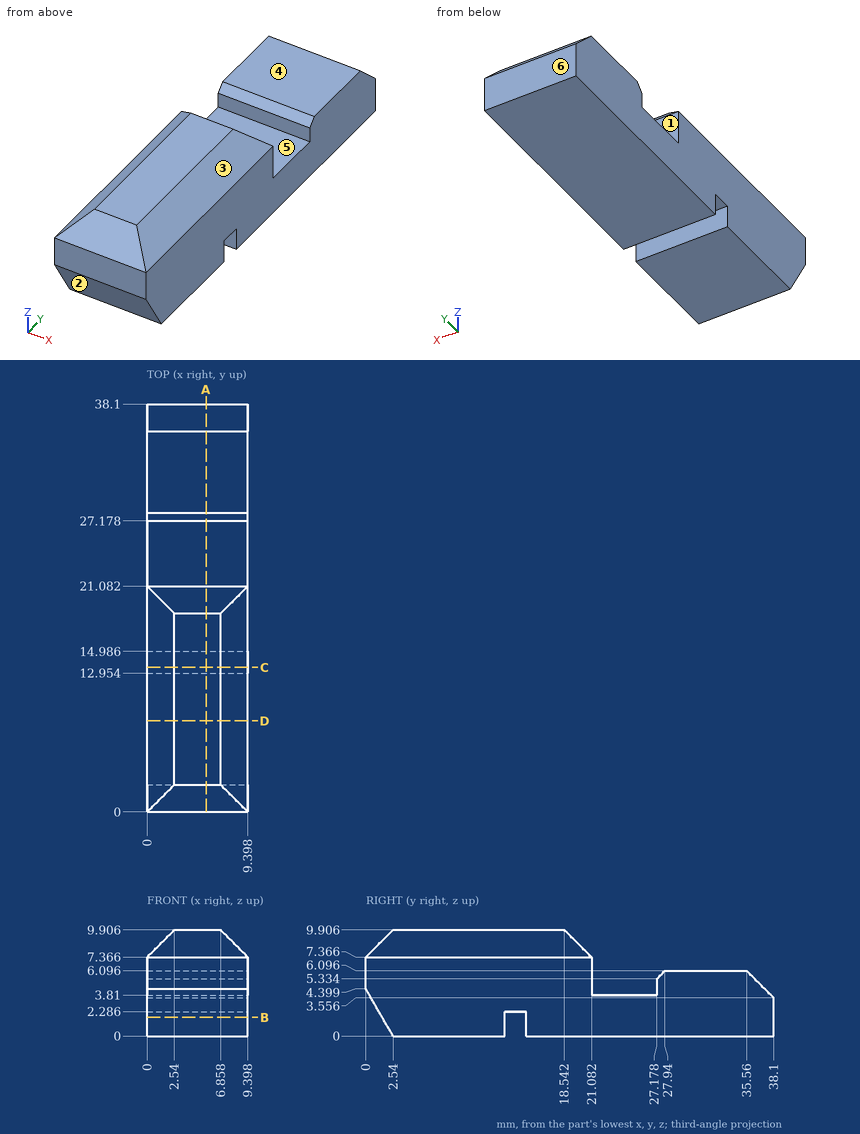
Verification items for this drawing (mm, ordinates from the low corner). A direction names the side the tool comes from. Coordinates: 2 decimals unless noted, no trailing zeros. Order: outer loops, then holes, each group sorted by start corner. A loop starts at its lowest first (then second) coordinate and runs counter-clockwise, first axis right, second up. Notation, with made-up numbers: M -11.5,61 L -2.5,61 A30 ccw -2.5,84 Z; hole C -23,58 d9. An arc over 180 degrees is marked long. One line per item, written item: value. Start each with the question number.
Item 1: Sectioned sample at D-D on y = 8.5. Record the cut outline in (x, z).
Item 2: Thickness scan on probe 1 along Y at (x, z) = (6.75, 6.75); probe 2 along Y at (x, z) = (5.5, 5) (1 decimal); probe 3 along Z at (x, y) = (8.5, 31). Record the ranges inside material, lowest first.
Item 3: Mould release check, pull along Y, two halves, no side actions. Record for the marked faces 1, 2 and 3: pulls with the +Y half, pulls with the -Y half, needs draft (parallel to the pull), parting line crosses it, or undercut.
Item 4: Sectioned sample at A-A on x = 5.5. Record the cut outline in (y, z).
Item 5: Sectioned sample at B-B on z = 1.75. Record the cut outline in (x, y).
Item 6: Sectioned sample at C-C on y = 13.5. Record the cut outline in (x, z).
Item 7: Depth check by flat-ended pin: P1, Ø0.6, axis at x = 2.5, y = 13.5, coming from the -Z side; P2, Ø3, axis at x = 6, y = 23.5, coming from the +Z side; P3, Ø4, axis at x = 1.5, y = 34.5, coming from the +Z side. Enter the tip coordinate at first touch or a pass-through.
Item 8: Access from +Z, -Z, +X, -X, +Y, -Y to the whole of each face (thin tool, end or side, straight path). Record for the marked faces 4, 5 and 6.
Calculated:
1. outline: M 0,0 L 9.4,0 L 9.4,7.37 L 6.86,9.91 L 2.54,9.91 L 0,7.37 Z
2. probe 1: 0 to 21.08
2. probe 2: 0 to 21.1, 27.2 to 36.7
2. probe 3: 0 to 6.1
3. face 1: undercut
3. face 2: pulls with the -Y half
3. face 3: needs draft
4. outline: M 0,4.4 L 2.54,0 L 12.95,0 L 12.95,2.29 L 14.99,2.29 L 14.99,0 L 38.1,0 L 38.1,3.56 L 35.56,6.1 L 27.94,6.1 L 27.18,5.33 L 27.18,3.81 L 21.08,3.81 L 21.08,7.37 L 18.54,9.91 L 2.54,9.91 L 0,7.37 Z
5. outline: M 0,1.53 L 9.4,1.53 L 9.4,12.95 L 0,12.95 Z; M 0,14.99 L 9.4,14.99 L 9.4,38.1 L 0,38.1 Z
6. outline: M 0,2.29 L 9.4,2.29 L 9.4,7.37 L 6.86,9.91 L 2.54,9.91 L 0,7.37 Z
7. P1: z = 2.29
7. P2: z = 3.81
7. P3: z = 6.1
8. face 4: +Z, +X, -X, +Y
8. face 5: +Z, +X, -X
8. face 6: +Z, -Z, +X, -X, +Y
